Read the model definition and answer for the solid it produces. Units are mm, in the model's axes. Give positions to 0.01 mm unless a question says otherwise; leave off trailing zeros. Write each loop counter-clockwise with the first axis right and the second up, starting at its lowest first coordinate (ties: lowest second). Pieces come first, ordered by that corner, then holes. Notation, with made-up numbers: M -9.5,48.25 L 24.5,48.25 A30 cw 24.5,86.25 Z; hole C -15,45.5 d8. An arc over 180 degrees is marked long. Use a Markdown table: item, result. Add a question column.
Item 1: The mould has two halves that part along X. Classify faces 1 (the flat face through (125, -13, 0)), 2 (the cylindrical face through (238.187, -12.522, 140.68)), 3 (the flat face through (0, -13, 75)): pulls with the +X half, pulls with the -X half, needs draft (parallel to the pull), parting line crosses it, or undercut.
Item 2: Consider probe 1 along Z at (x, y) = (12.7, -18.5); probe 2 along Z at (x, y) = (239, -2.5); probe 3 along X at (y, z) = (-22, 63). Determine where each line is inside the solid, lowest interval first. Write a range as [from, to].
Item 3: A cutting plane is placed at C-C on y = -9.5. Determine the outline of the cut face in (x, z), then the cut area to 3 significant figures.
Item 4: A cutting plane is placed at A-A on z = 76.2. Determine the outline of the cut face in (x, y).
Item 5: A cutting plane is placed at D-D on z = 12.7. Determine the outline of the cut face in (x, y), then the cut area to 3 significant figures.
Item 6: A cutting plane is placed at B-B on x = 127. Determine the outline of the cut face in (y, z).
from build123d import *

# Parameters (mm, degrees)
F0_W     = 254
F0_H     = 152.4
F1_DEPTH = 25.4
F3_D     = 6.5278
F4_R     = 28.401981162
F5_DEPTH = 25.401


with BuildPart() as f1:
    # F0 (on Front) → F1 (new body)
    with BuildSketch(Plane.XZ):
        with Locations((127, 76.2)):
            Rectangle(F0_W, F0_H)
    extrude(amount=F1_DEPTH)

    # F3 (through all)
    with Locations(Plane.XZ.offset(25.4)):
        with Locations((12.7, 139.7), (241.3, 139.7), (241.3, 12.7), (12.7, 12.7)):
            Hole(F3_D / 2)

    # F4 (on face) → F5 (cut, through all)
    with BuildSketch(Plane(origin=(0, 0, 0), x_dir=(-1, 0, 0), z_dir=(0, 1, 0))):
        with Locations((-127, 76.2)):
            Circle(F4_R)
    extrude(amount=-F5_DEPTH, mode=Mode.SUBTRACT)


solid = f1.part
Filled in:
| question | item | result |
|---|---|---|
| 1 | face 1 | needs draft |
| 1 | face 2 | undercut |
| 1 | face 3 | pulls with the -X half |
| 2 | probe 1 | [0, 9.44], [15.96, 136.44], [142.96, 152.4] |
| 2 | probe 2 | [0, 10.38], [15.02, 137.38], [142.02, 152.4] |
| 2 | probe 3 | [0, 101.85], [152.15, 254] |
| 3 | outline | M 0,0 L 254,0 L 254,152.4 L 0,152.4 Z; hole C 12.7,12.7 d6.53; hole C 12.7,139.7 d6.53; hole C 127,76.2 d56.8; hole C 241.3,12.7 d6.53; hole C 241.3,139.7 d6.53 |
| 3 | area | 36,000 mm² |
| 4 | outline | M 0,-25.4 L 98.6,-25.4 L 98.6,0 L 0,0 Z; M 155.4,-25.4 L 254,-25.4 L 254,0 L 155.4,0 Z |
| 5 | outline | M 0,-25.4 L 9.44,-25.4 L 9.44,0 L 0,0 Z; M 15.96,-25.4 L 238.04,-25.4 L 238.04,0 L 15.96,0 Z; M 244.56,-25.4 L 254,-25.4 L 254,0 L 244.56,0 Z |
| 5 | area | 6,120 mm² |
| 6 | outline | M -25.4,0 L 0,0 L 0,47.8 L -25.4,47.8 Z; M -25.4,104.6 L 0,104.6 L 0,152.4 L -25.4,152.4 Z |
